The model under review builds one solid part; all positions refer to its coordinate system, in mm. Face numbers are marked on the shaded views. A direction names the side the tool comes from. Coordinates: 2 decimals unless noted, no trailing zeros. Loops run counter-clockwise (first coordinate to the right, second up) from the corner with the lowest first, then second, coordinate; pieces in that order, holes last. Notation, with made-up numbers: M 80,3 L 127,3 A13 ccw 127,15 Z; hole C 55.25,79 d2. An arc over 180 degrees is marked long. One line per item, written item: value.
```python
from build123d import *

# Parameters (mm, degrees)
F0_W     = 100
F0_H     = 100
F1_DEPTH = 100
F2_W     = 143.886555
F2_H     = 64.474793
F3_DEPTH = 48
F4_R     = 2.5
F5_DEPTH = 52.001
F6_W     = 124.598865
F6_H     = 122.024197
F7_DEPTH = 25


with BuildPart() as f1:
    # F0 (on Top) → F1 (new body)
    with BuildSketch(Plane.XY):
        with Locations((4.466346, 18.817768)):
            Rectangle(F0_W, F0_H)
    extrude(amount=F1_DEPTH)

    # F2 (on face) → F3 (cut)
    with BuildSketch(Plane.XY.offset(100)):
        with Locations((11.580882, -6.759453)):
            Rectangle(F2_W, F2_H)
    extrude(amount=-F3_DEPTH, mode=Mode.SUBTRACT)

    # F4 (on face) → F5 (cut, through all)
    with BuildSketch(Plane.XY.offset(52)):
        with Locations((-3.175375, 0)):
            Circle(F4_R)
    extrude(amount=-F5_DEPTH, mode=Mode.SUBTRACT)

    # F6 (on face) → F7 (cut)
    with BuildSketch(Plane(origin=(0, 0, 0), x_dir=(1, 0, 0), z_dir=(0, 0, -1))):
        with Locations((3.516642, -17.77996)):
            Rectangle(F6_W, F6_H)
    extrude(amount=-F7_DEPTH, mode=Mode.SUBTRACT)


solid = f1.part
```
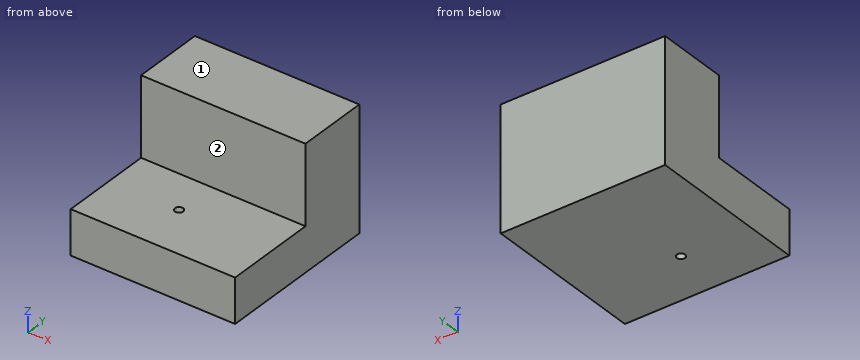
(1) Insertion check: pin 1 Ø5 at (x, y) = (-27.5, -1) entering from +Z; pin 2 Ø14.5 at (x, z) = (25, 80) entering from -Y. Each pin has a flat end and moves straight along its axis. Give the tip position at first contact, or say it passes through.
Checks:
pin 1: z = 52
pin 2: y = 25.48
(2) Add section B-B on x = 29.5. State the section outline as (y, z) points, then the cut area to 3 significant figures.
Checks:
outline: M -31.18,25 L 68.82,25 L 68.82,100 L 25.48,100 L 25.48,52 L -31.18,52 Z
area: 4,780 mm^2
(3) Add section D-D on y = -22.5. State the section outline as (x, z) points.
Checks:
outline: M -45.53,25 L 54.47,25 L 54.47,52 L -45.53,52 Z
(4) Add section C-C on z = 70. State the section outline as (x, y) points.
Checks:
outline: M -45.53,25.48 L 54.47,25.48 L 54.47,68.82 L -45.53,68.82 Z
(5) Add section A-A on y = 0. State the section outline as (x, z) points, then the cut area to 4 significant figures.
Checks:
outline: M -45.53,25 L -5.68,25 L -5.68,52 L -45.53,52 Z; M -0.68,25 L 54.47,25 L 54.47,52 L -0.68,52 Z
area: 2,565 mm^2
(6) To check wall thickness, follow L1, parallel to Y at x = -4, z = 57.5; L2, parallel to Z at x = 10, y = 20. State the ranges of each line that lie inside material, in increasing order. Write a range as [from, to].
Checks:
L1: [25.48, 68.82]
L2: [25, 52]
(7) Tool access review of the marked faces 1 and 2: name each direction out of +Z, -Z, +X, -X, +Y, -Y from which nothing blocks a thin tool from reaching the whole face with its end or side.
Checks:
face 1: +Z, +X, -X, +Y, -Y
face 2: +Z, +X, -X, -Y
